The listing builds one solid part. Answer for the finished solid, in the listing's coordinates (mm). Face numbers are marked on the shaded views. A direction names the side the tool comes from. Coordinates: 2 decimals unless noted, no trailing zeros. Order: outer loops, then holes, each group sorted by start corner. A loop starts at its lowest first (then second) coordinate and runs counter-clockwise, first axis right, second up.
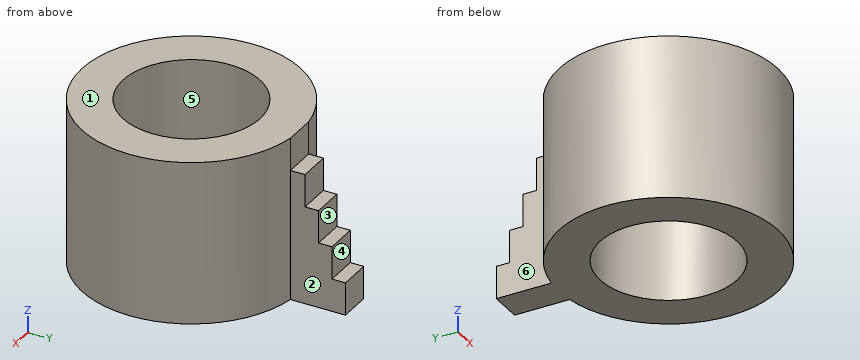
from build123d import *

# Parameters (mm, degrees)
F0_R     = 10.668
F1_DEPTH = 25.4
F3_DEPTH = 12.7


with BuildPart() as f1:
    # F0 (on Top) → F1 (new body)
    with BuildSketch(Plane.XY):
        with BuildLine():
            Line((-2.54, 25.4), (-2.54, 16.8273801883))
            ThreePointArc((-2.54, 16.8273801883), (0, -17.018), (2.54, 16.8273801883))
            Line((2.54, 16.8273801883), (2.54, 25.4))
            Line((2.54, 25.4), (-2.54, 25.4))
        make_face()
        Circle(F0_R, mode=Mode.SUBTRACT)
    extrude(amount=F1_DEPTH)

    # F2 (on Right) → F3 (cut, symmetric)
    with BuildSketch(Plane.YZ):
        Polygon((23.3045, 5.08), (25.4, 5.08), (25.4, 0), (25.4, -8.07502307), (34.9588990211, -8.07502307), (34.9588990211, 29.4091364962), (16.8273801883, 29.4091364962), (16.8273801883, 20.32), (19.1135, 20.32), (19.1135, 15.24), (21.209, 15.24), (21.209, 10.16), (23.3045, 10.16), align=None)
    extrude(amount=F3_DEPTH, both=True, mode=Mode.SUBTRACT)


solid = f1.part
(1) Find section D-D on y = 7.5. Determine the outline of the cut face in (x, z).
(2) Find the intervals of material crossed by probe 1 along X at (y, z) = (0.5, 7.5); probe 2 along X at (y, z) = (-3.5, 11.5); probe 3 along Z at (x, y) = (-1, 23), in increasing order.
(3) A tool of negligible diameter and unlimited length cuts with its end or side. For the marked faces 1, 2 and 3, from which of +Z, -Z, +X, -X, +Y, -Y can it reach the whole face along a straight path? Write none if from no direction.
(4) Given pin 1 Ø12 at (y, z) = (7, 10.5) entering from -X; pin 2 Ø5.5 at (x, z) = (0, 11.5) entering from +Y; pin 3 Ø12 at (x, z) = (1, 20) entering from +Y; pin 4 Ø12 at (x, y) = (-1.5, 18) entering from +Z, each flat-ended and moving along its own axis, determine where each tip first touches the part or whether it passes through.
(5) Find section A-A on y = 0. Determine the outline of the cut face in (x, z), then the cut area to 3 significant figures.
(6) The mould has two halves that part along Y. Classify the marked faces 4, 5 and 6: pulls with the +Y half, pulls with the -Y half, needs draft (parallel to the pull), parting line crosses it, or undercut.
(7) Find section C-C on x = 0. Determine the outline of the cut face in (y, z), then the cut area to 3 significant figures.
(8) Find section B-B on z = 18.5. Determine the outline of the cut face in (x, y).
Resolved:
1. outline: (-15.28, 0) - (-7.59, 0) - (-7.59, 25.4) - (-15.28, 25.4) - close; (7.59, 0) - (15.28, 0) - (15.28, 25.4) - (7.59, 25.4) - close
2. probe 1: x = -17.01 to -10.66, 10.66 to 17.01
2. probe 2: x = -16.65 to -10.08, 10.08 to 16.65
2. probe 3: z = 0 to 10.16
3. face 1: +Z, +X, -X, +Y, -Y
3. face 2: +Z, -Z, +X, +Y
3. face 3: +Z, +X, -X, +Y
4. pin 1: stops at x = -16.99
4. pin 2: stops at y = 23.3
4. pin 3: stops at y = 21.21
4. pin 4: stops at z = 25.4
5. outline: (-17.02, 0) - (-10.67, 0) - (-10.67, 25.4) - (-17.02, 25.4) - close; (10.67, 0) - (17.02, 0) - (17.02, 25.4) - (10.67, 25.4) - close
5. area: 323 mm2
6. face 4: pulls with the +Y half
6. face 5: undercut
6. face 6: needs draft
7. outline: (-17.02, 0) - (-10.67, 0) - (-10.67, 25.4) - (-17.02, 25.4) - close; (10.67, 0) - (25.4, 0) - (25.4, 5.08) - (23.3, 5.08) - (23.3, 10.16) - (21.21, 10.16) - (21.21, 15.24) - (19.11, 15.24) - (19.11, 20.32) - (16.83, 20.32) - (16.83, 25.4) - (10.67, 25.4) - close
7. area: 428 mm2
8. outline: (-2.54, 16.83) arc R17.02 ccw (long way) to (2.54, 16.83) - (2.54, 19.11) - (-2.54, 19.11) - close; hole circle Ø21.34 at (0, 0)
